Can you work these out from the model? Positions are in its coordinate system, mm. Give positions to 0.01 mm unless a question says otherwise; leave off trailing zeros. Order: outer loops, then holes, each group sorted by start corner. A loop starts at its lowest first (then second) coordinate and runs counter-clockwise, first axis right, second up. Notation, with made-up numbers: (56, 3.25) - (90, 3.25) arc R9 cw to (90, 17.25) - close; hole circle Ø8 at (30, 40.5). An arc over 180 degrees is marked (long way). Answer as a JSON object with one key per item and string values.
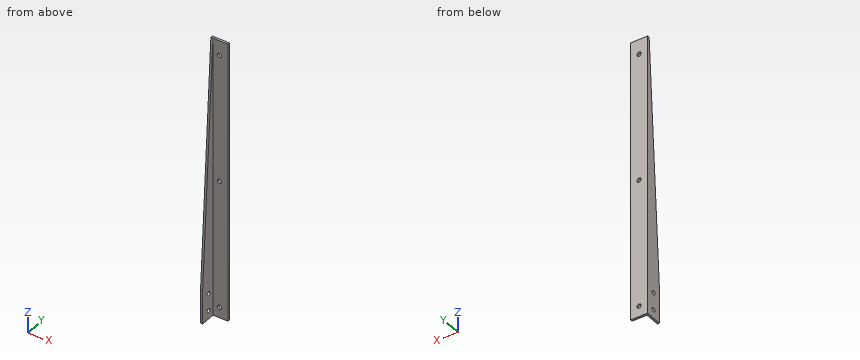
Autodesk Inventor part; units mm, degrees
ref_plane "YZ Plane" through (0, 0, 0) normal (1, 0, 0) x (0, 1, 0)
ref_plane "XZ Plane" through (0, 0, 0) normal (0, 1, 0) x (-1, 0, 0)
ref_plane "XY Plane" through (0, 0, 0) normal (0, 0, 1) x (1, 0, 0)
sketch "Sketch1" plane through (0, 0, 0) normal (0, 0, 1) x (1, 0, 0)
  line L0 (0, 0) -> (25.4, 0)
  line L1 (25.4, 0) -> (25.4, -3.175)
  line L2 (25.4, -3.175) -> (0, -3.175)
  line L3 (0, -3.175) -> (0, 0)
  line L4 (0, 0) -> (3.175, 0)
  line L5 (3.175, 0) -> (3.175, -25.4)
  line L6 (3.175, -25.4) -> (0, -25.4)
  line L7 (0, -25.4) -> (0, 0)
  dimension "d0" = 25.4
  dimension "d1" = 3.175
  dimension "d2" = 3.175
  dimension "d3" = 25.4
extrude "Extrusion1" add sketch "Sketch1" along normal blind 419.1
sketch "Sketch2" plane through (0, -25.4, 0) normal (-1, 0, 0) x (0, 0, 1)
  line L0 (419.1, 25.4) -> (419.1, 0)
  line L1 (0, 25.4) -> (419.1, 25.4)
  line L2 (0, 25.4) -> (0, 0)
  line L3 (0, 0) -> (419.1, 0)
  line L4 (0, 0) -> (50.8, 0) construction
  line L5 (0, 0) -> (419.1, 0) construction
  line L6 (419.1, 25.4) -> (419.1, 22.225) construction
  line L7 (419.1, 0) -> (419.1, 22.225) construction
  line L8 (419.1, 22.225) -> (50.8, 0)
  line L9 (50.8, 0) -> (419.1, 0)
  line L10 (419.1, 22.225) -> (0, 22.225)
  line L11 (419.1, 0) -> (419.1, 22.225)
  dimension "d6" = 50.8
  dimension "d7" = 3.175
extrude "Extrusion2" cut sketch "Sketch2" against normal blind 431.8 contours L0 L3 L8
sketch "Sketch3" plane through (0, -25.4, 0) normal (-1, 0, 0) x (0, 0, 1)
  line L0 (50.8, 0) -> (419.1, 22.225)
  line L1 (419.1, 25.4) -> (419.1, 22.225)
  line L2 (0, 25.4) -> (419.1, 25.4)
  line L3 (0, 25.4) -> (0, 0)
  line L4 (0, 0) -> (50.8, 0)
  point P0 (12.7, 12.7)
  point P1 (38.1, 12.7)
  dimension "d10" = 12.7
  dimension "d11" = 12.7
  dimension "d12" = 38.1
  dimension "d13" = 12.7
hole "Hole1" at (0, -12.7, 12.7) at (0, -12.7, 38.1) direction (1, 0, 0) diameter 6.35 end through all
sketch "Sketch4" plane through (0, 0, 0) normal (0, 1, 0) x (1, 0, 0)
  line L0 (25.4, 0) -> (0, 0)
  line L1 (0, 0) -> (0, -419.1)
  line L2 (25.4, -419.1) -> (0, -419.1)
  line L3 (25.4, 0) -> (25.4, -419.1)
  point P0 (12.7, -15.875)
  point P1 (12.7, -206.375)
  point P2 (12.7, -396.875)
  dimension "d21" = 12.7
  dimension "d22" = 15.875
  dimension "d23" = 206.375
  dimension "d24" = 12.7
  dimension "d25" = 12.7
  dimension "d26" = 22.225
hole "Hole2" at (12.7, 0, 15.875) at (12.7, 0, 206.375) at (12.7, 0, 396.875) direction (0, -1, 0) diameter 6.35 end through all
properties part number "1x1 lengthwise left"
Q1. I'm going to push flat-ended pins straight in: pin 1 Ø8 at (x, z) = (13.5, 221.5) entering from +Y; pin 2 Ø10 at (x, z) = (12.7, 396.875) entering from -Y (3 decimals); pin 3 Ø6 at (y, z) = (-7.5, 322.5) entering from +X (3 decimals). Where does each tip first touch, or does it pass through?
Recorded:
{"pin 1": "stops at y = 0", "pin 2": "stops at y = -3.175", "pin 3": "stops at x = 3.175"}
Q2. If we section it at B-B, the plane y = -20.75: Please give me the cut outline in (x, z) (3 decimals), then the cut area to 3 significant figures.
Recorded:
{"outline": "(0, 0) - (3.175, 0) - (3.175, 127.857) - (0, 127.857) - close", "area": "406 mm^2"}
Q3. I need wall thicknesses on L1, parallel to Z at x = 12.7, y = -1.35; L2, parallel to X at y = -4, z = 348.5 (3 decimals); L3, parallel to Y at x = 23, z = 396.5 (3 decimals). Which ranges of each line are inside material? Lowest first, please.
Recorded:
{"L1": "z = 0 to 12.7, 19.05 to 203.2, 209.55 to 393.7, 400.05 to 419.1", "L2": "x = 0 to 3.175", "L3": "y = -3.175 to 0"}
Q4. If we section it at A-A, the plane z = 103: Please give me the cut outline in (x, y) (3 decimals).
Recorded:
{"outline": "(0, -22.25) - (3.175, -22.25) - (3.175, -3.175) - (25.4, -3.175) - (25.4, 0) - (0, 0) - close"}
Q5. If we section it at C-C, the plane z = 180: Please give me the cut outline in (x, y) (3 decimals).
Recorded:
{"outline": "(0, -17.603) - (3.175, -17.603) - (3.175, -3.175) - (25.4, -3.175) - (25.4, 0) - (0, 0) - close"}
